The listing builds one solid part. Answer for the finished solid, in the listing's coordinates (mm). Round coordinates to 2 decimals unless told otherwise and drop trailing zeros. Write each loop counter-clockwise with the first axis right and the second up, starting at its lowest first coordinate (ties: lowest second). Pieces come first, ordered by that corner, then holes.
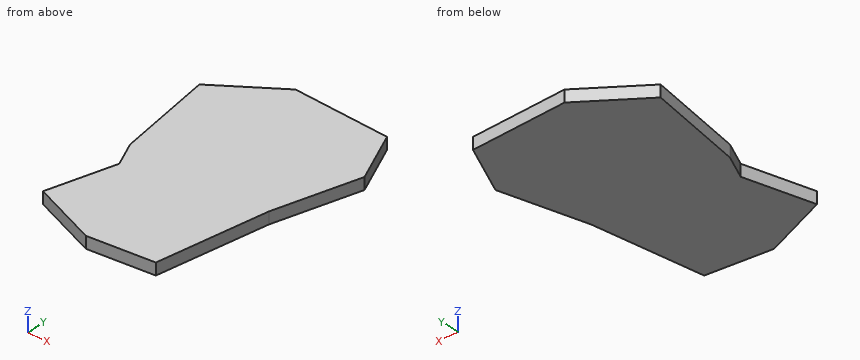
Autodesk Inventor part; units mm, degrees
ref_plane "YZ Plane" through (0, 0, 0) normal (1, 0, 0) x (0, 1, 0)
ref_plane "XZ Plane" through (0, 0, 0) normal (0, 1, 0) x (-1, 0, 0)
ref_plane "XY Plane" through (0, 0, 0) normal (0, 0, 1) x (1, 0, 0)
sketch "Sketch1" plane through (0, 0, 0) normal (0, 0, 1) x (1, 0, 0)
  line L0 (-15.9123, 14.7509) -> (784.1877, 14.7509) construction
  line L1 (784.1877, 14.7509) -> (784.1877, -1052.0491) construction
  line L2 (784.1877, -1052.0491) -> (-15.9123, -1052.0491) construction
  line L3 (-15.9123, -1052.0491) -> (-15.9123, 14.7509) construction
  line L4 (311.9145, -258.6605) -> (525.4879, -272.6195)
  line L5 (525.4879, -272.6195) -> (581.2504, -393.4383)
  line L6 (581.2504, -393.4383) -> (533.62, -580.4751)
  line L7 (533.62, -580.4751) -> (498.7684, -826.7595)
  line L8 (498.7684, -826.7595) -> (355.243, -838.8475)
  line L9 (355.243, -838.8475) -> (208.3043, -778.5549)
  line L10 (208.3043, -778.5549) -> (246.337, -629.207)
  line L11 (246.337, -629.207) -> (219.57, -571.2118)
  line L12 (219.57, -571.2118) -> (180.7596, -351.4058)
  line L13 (180.7596, -351.4058) -> (311.9145, -258.6605)
  line L14 (180.7596, -258.6605) -> (584.1903, -258.6605)
  line L15 (584.1903, -258.6605) -> (584.1903, -838.8475)
  line L16 (584.1903, -838.8475) -> (180.7596, -838.8475)
  line L17 (180.7596, -838.8475) -> (180.7596, -258.6605)
  point P0 (0, 0)
  dimension "d7" = 403.4308
  dimension "d10" = 580.187
extrude "Extrusion1" add sketch "Sketch1" against normal blind 25.4 contours L4 L5 L6 L7 L8 L9 L10 L11 L12 L13
properties part number "emu"
1. Section B-B on y = -442.5 is taken. Determine the outline of the cut face in (x, z), plus the area to 3 significant figures.
Geometry says:
outline: (196.84, -25.4) - (568.76, -25.4) - (568.76, 0) - (196.84, 0) - close
area: 9,450 mm2
2. Section C-C on x = 298.5 is taken. Determine the outline of the cut face in (y, z), plus the area to 3 significant figures.
Geometry says:
outline: (-815.56, -25.4) - (-268.15, -25.4) - (-268.15, 0) - (-815.56, 0) - close
area: 13,900 mm2
3. Section A-A on z = -13 is taken. Determine the outline of the cut face in (x, y), plus the area to 3 significant figures.
Geometry says:
outline: (180.76, -351.41) - (219.57, -571.21) - (246.34, -629.21) - (208.3, -778.55) - (355.24, -838.85) - (498.77, -826.76) - (533.62, -580.48) - (581.25, -393.44) - (525.49, -272.62) - (311.91, -258.66) - close
area: 178,000 mm2
4. Given pin 1 (5 mm diameter, centred on x = 273, z = -9.5, fed in from -Y); pin 2 (10 mm diameter, centred on y = -602, z = -22.5, fed in from -X); pin 3 (4 mm diameter, centred on y = -618, z = -14.5, fed in from +X), each flat-ended and moving along its own axis, determine where each tip first touches the part or whether it passes through.
Geometry says:
pin 1: stops at y = -806.13
pin 2: stops at x = 231.47
pin 3: stops at x = 528.59
5. Straight lines are drawn through the part: line 1 along Y through (x, z) = (453, -8); line 2 along X through (y, z) = (-353, -11.75); line 3 along X through (y, z) = (-511.5, -13.25). For each, find the intervals that lie inside material, in ascending order.
Geometry says:
line 1: y = -830.61 to -267.88
line 2: x = 181.04 to 562.59
line 3: x = 209.03 to 551.19
